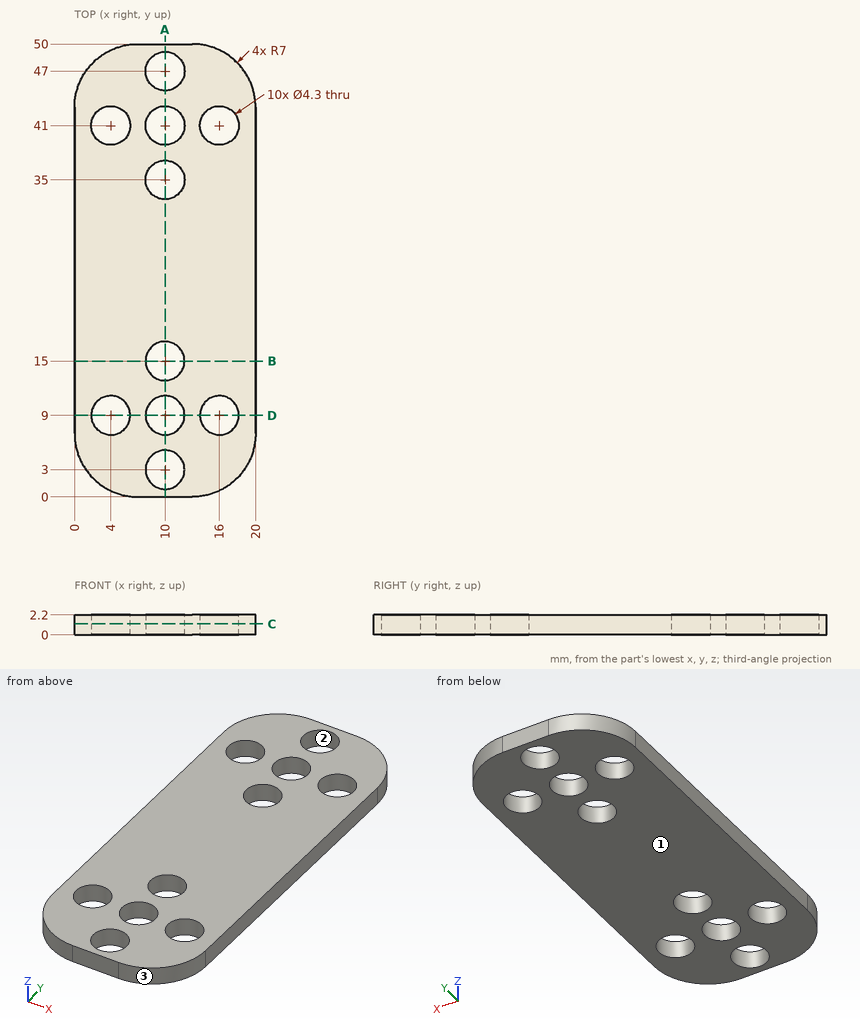
Print and shaded views of the part. All mm, measured from the part's lowest x, y and z. Round coordinates to 2 decimals unless told otherwise and drop trailing zeros. Write each loop counter-clockwise with the first axis right and the second up, starting at its lowest first coordinate (ties: lowest second). Pieces come first, ordered by that corner, then holes. Notation, with made-up numbers: M -30.75,68.5 L -6.75,68.5 A33 cw -6.75,107.5 Z; hole C 81,85 d8. An arc over 180 degrees is marked long. One line per question, with ' | ' between items.
(1) Two-plate mould, pull along Y, no slides. Class the marked faces 1, 2 and 3: released by +Y, released by -Y, zero draft, split by the parting line, or undercut.
Answer key:
face 1: zero draft | face 2: undercut | face 3: released by -Y
(2) Saw through at C-C on z = 1.2. Count the separate pieces of the cut face and the enclosed holes in it, then the cut area to 3 significant figures.
Answer key:
separate pieces: 1 | enclosed holes: 10 | area: 813 mm^2
(3) Probe line 1 along X through (y, z) = (41, 1.45); line 2 along X through (y, z) = (10.5, 1.4); line 3 along Y through (x, z) = (16, 0.8). List the from-to ranges inside material, lowest first.
Answer key:
line 1: x = 0 to 1.85, 6.15 to 7.85, 12.15 to 13.85, 18.15 to 20 | line 2: x = 0 to 2.46, 5.54 to 8.46, 11.54 to 14.46, 17.54 to 20 | line 3: y = 0.68 to 6.85, 11.15 to 38.85, 43.15 to 49.32
(4) Saw through at B-B on y = 15. Write the cut outline in (x, z), then the cut area to 3 significant figures.
Answer key:
outline: M 0,0 L 7.85,0 L 7.85,2.2 L 0,2.2 Z; M 12.15,0 L 20,0 L 20,2.2 L 12.15,2.2 Z | area: 34.5 mm^2
(5) Saw through at A-A on x = 10. Write the cut outline in (y, z), then the cut area to 3 significant figures.
Answer key:
outline: M 0,0 L 0.85,0 L 0.85,2.2 L 0,2.2 Z; M 5.15,0 L 6.85,0 L 6.85,2.2 L 5.15,2.2 Z; M 11.15,0 L 12.85,0 L 12.85,2.2 L 11.15,2.2 Z; M 17.15,0 L 32.85,0 L 32.85,2.2 L 17.15,2.2 Z; M 37.15,0 L 38.85,0 L 38.85,2.2 L 37.15,2.2 Z; M 43.15,0 L 44.85,0 L 44.85,2.2 L 43.15,2.2 Z; M 49.15,0 L 50,0 L 50,2.2 L 49.15,2.2 Z | area: 53.2 mm^2
(6) Saw through at D-D on y = 9. Write the cut outline in (x, z).
Answer key:
outline: M 0,0 L 1.85,0 L 1.85,2.2 L 0,2.2 Z; M 6.15,0 L 7.85,0 L 7.85,2.2 L 6.15,2.2 Z; M 12.15,0 L 13.85,0 L 13.85,2.2 L 12.15,2.2 Z; M 18.15,0 L 20,0 L 20,2.2 L 18.15,2.2 Z
(7) Pin check, flat tip, straight feed: pin 1 (3.5 mm diameter, centred on x = 16, y = 9, fed in from -Z). Stop position of the tip, or through.
Answer key:
pin 1: passes through
